The model under review builds one solid part; all positions refer to its coordinate system, in mm. A direction names the side the tool comes from. Round coordinates to 2 decimals unless told otherwise and drop trailing zeros. Loops run counter-clockwise (first coordinate to the right, second up) from the corner with the lowest first, then second, coordinate; pieces in that order, holes last. Notation, with made-up numbers: (51.25, 6.25) -> (58.25, 6.25) arc R20 ccw to (58.25, 39.25) -> close; hole circle Ø2 at (61.25, -3.5). An arc over 180 degrees is marked (long way). Use a Markdown table: item, result. Add a question column.
1) Wall thickness on probe 1 along X at (y, z) = (82.5, 14.5); probe 2 along Y at (x, z) = (207.5, 1.25): over which ranges is each line inside the solid? List them lowest first.
2) Mouldability with a two-part tool opening along Y and no side actions: class faces 1 (the flat face through (177, 441.642, 13)), 2 (the flat face through (-60.823, 184, 13)), 3 (the flat face through (434.477, 184, 13)), 4 (the flat face through (177, 428.942, 13)) as released by +Y, released by -Y, zero draft, split by the parting line, or undercut.
3) Consider section A-A on x = 270.5. Give the boundary of the cut face in (y, z), plus the area to 3 significant figures.
4) Consider section B-B on y = 241.5. Give the boundary of the cut face in (x, z), plus the area to 3 significant figures.
5) For faces 5 (the flat face through (421.777, 184, 13)), 6 (the flat face through (-73.523, 184, 13)), list the 3-axis set-ups (+Z, -Z, +X, -X, +Y, -Y) from which the entire face can be reached by the end or side of a thin tool; tool diameter is ignored.
6) Consider section C-C on z = 12. Give the boundary of the cut face in (x, y), plus the area to 3 significant figures.
from build123d import *

# Parameters (mm, degrees)
F0_W     = 508
F0_H     = 508
F1_DEPTH = 25.4
F2_T     = -12.7
F3_DEPTH = 1396.1044084281


with BuildPart() as f1:
    # F0 (on Top) → F1 (new body)
    with BuildSketch(Plane.XY):
        with Locations((180.4774918556, 187.6424022913)):
            Rectangle(F0_W, F0_H)
    extrude(amount=F1_DEPTH)

    # F2
    f2_openings = [f1.faces().sort_by_distance(p)[0] for p in [
        (180.477492, 187.642402, 25.4),
    ]]
    offset(amount=F2_T, openings=f2_openings)

    # F3 (cut): a face of the model
    f3_faces = [f1.faces().sort_by_distance(p)[0] for p in [
        (180.4774918556, 187.6424022913, 12.7),
    ]]
    extrude(f3_faces, amount=-F3_DEPTH, mode=Mode.SUBTRACT)


solid = f1.part
Result set:
| question | item | result |
|---|---|---|
| 1 | probe 1 | -73.52 to -60.82, 421.78 to 434.48 |
| 1 | probe 2 | -66.36 to -53.66, 428.94 to 441.64 |
| 2 | face 1 | released by +Y |
| 2 | face 2 | undercut |
| 2 | face 3 | zero draft |
| 2 | face 4 | undercut |
| 3 | outline | (-66.36, 0) -> (-53.66, 0) -> (-53.66, 25.4) -> (-66.36, 25.4) -> close; (428.94, 0) -> (441.64, 0) -> (441.64, 25.4) -> (428.94, 25.4) -> close |
| 3 | area | 645 mm2 |
| 4 | outline | (-73.52, 0) -> (-60.82, 0) -> (-60.82, 25.4) -> (-73.52, 25.4) -> close; (421.78, 0) -> (434.48, 0) -> (434.48, 25.4) -> (421.78, 25.4) -> close |
| 4 | area | 645 mm2 |
| 5 | face 5 | +Z, -Z |
| 5 | face 6 | +Z, -Z, -X, +Y, -Y |
| 6 | outline | (-73.52, -66.36) -> (434.48, -66.36) -> (434.48, 441.64) -> (-73.52, 441.64) -> close; hole (-60.82, -53.66) -> (421.78, -53.66) -> (421.78, 428.94) -> (-60.82, 428.94) -> close |
| 6 | area | 25,200 mm2 |
